from build123d import *

# Parameters (mm, degrees)
EXTRUDE_1_DEPTH     = 5
SKETCH_2_R          = 1.25
CUT_EXTRUDE_1_DEPTH = 7.5
SKETCH_3_R          = 1.25
CUT_EXTRUDE_2_DEPTH = 7.5
SKETCH_4_R          = 1.25
CUT_EXTRUDE_3_DEPTH = 76.013332148
SKETCH_5_R          = 0.75
CUT_EXTRUDE_4_DEPTH = 76.013332148
SKETCH_7_R          = 1.5
CUT_EXTRUDE_6_DEPTH = 76.013332148


with BuildPart() as part:
    # ｽｹｯﾁ1 → ﾎﾞｽ - 押し出し1 (new body)
    with BuildSketch(Plane.XY):
        Polygon((-29, 51), (-29, 0), (-23, 0), (-23, -3), (23, -3), (23, 0), (29, 0), (29, 51), (23, 51), (23, 59), (17, 59), (17, 69), (-17, 69), (-17, 59), (-23, 59), (-23, 51), align=None)
    extrude(amount=EXTRUDE_1_DEPTH)

    # ｽｹｯﾁ2 → ｶｯﾄ - 押し出し1 (cut)
    with BuildSketch(Plane(origin=(0, 59, 0), x_dir=(1, 0, 0), z_dir=(0, 1, 0))):
        with Locations(Location((-20, -2.5, 0), (0, 0, 270))):
            Circle(SKETCH_2_R)
        with Locations(Location((20, -2.5, 0), (0, 0, 270))):
            Circle(SKETCH_2_R)
    extrude(amount=-CUT_EXTRUDE_1_DEPTH, mode=Mode.SUBTRACT)

    # ｽｹｯﾁ3 → ｶｯﾄ - 押し出し2 (cut)
    with BuildSketch(Plane(origin=(0, 51, 0), x_dir=(1, 0, 0), z_dir=(0, 1, 0))):
        with Locations(Location((-26, -2.5, 0), (0, 0, 270))):
            Circle(SKETCH_3_R)
        with Locations(Location((26, -2.5, 0), (0, 0, 270))):
            Circle(SKETCH_3_R)
    cut_extrude_2 = extrude(amount=-CUT_EXTRUDE_2_DEPTH, mode=Mode.SUBTRACT)

    # ﾐﾗｰ1: ｶｯﾄ - 押し出し2 across plane
    add(cut_extrude_2.mirror(Plane.ZX.offset(25.5)), mode=Mode.SUBTRACT)

    # ｽｹｯﾁ4 → ｶｯﾄ - 押し出し3 (cut, through all)
    with BuildSketch(Plane(origin=(0, 0, 0), x_dir=(-1, 0, 0), z_dir=(0, 0, -1))):
        with Locations((-14.5, 66.5)):
            Circle(SKETCH_4_R)
        with Locations((14.5, 66.5)):
            Circle(SKETCH_4_R)
    extrude(amount=-CUT_EXTRUDE_3_DEPTH, mode=Mode.SUBTRACT)

    # ｽｹｯﾁ5 → ｶｯﾄ - 押し出し4 (cut, through all)
    with BuildSketch(Plane(origin=(0, 0, 0), x_dir=(-1, 0, 0), z_dir=(0, 0, -1))):
        with Locations((-17, 59)):
            Circle(SKETCH_5_R)
        with Locations((-23, 51)):
            Circle(SKETCH_5_R)
        with Locations((-23, 0)):
            Circle(SKETCH_5_R)
        with Locations((17, 59)):
            Circle(SKETCH_5_R)
        with Locations((23, 51)):
            Circle(SKETCH_5_R)
        with Locations((23, 0)):
            Circle(SKETCH_5_R)
    extrude(amount=-CUT_EXTRUDE_4_DEPTH, mode=Mode.SUBTRACT)

    # ｽｹｯﾁ7 → ｶｯﾄ - 押し出し6 (cut, through all)
    with BuildSketch(Plane.XY.offset(5)):
        with Locations((-26, 44)):
            Circle(SKETCH_7_R)
        with Locations(Location((-26, 7, 0), (0, 0, 180))):
            Circle(SKETCH_7_R)
        with Locations((-20, 52)):
            Circle(SKETCH_7_R)
        with Locations(Location((20, 52, 0), (0, 0, 180))):
            Circle(SKETCH_7_R)
        with Locations((26, 7)):
            Circle(SKETCH_7_R)
        with Locations(Location((26, 44, 0), (0, 0, 180))):
            Circle(SKETCH_7_R)
    extrude(amount=-CUT_EXTRUDE_6_DEPTH, mode=Mode.SUBTRACT)


solid = part.part
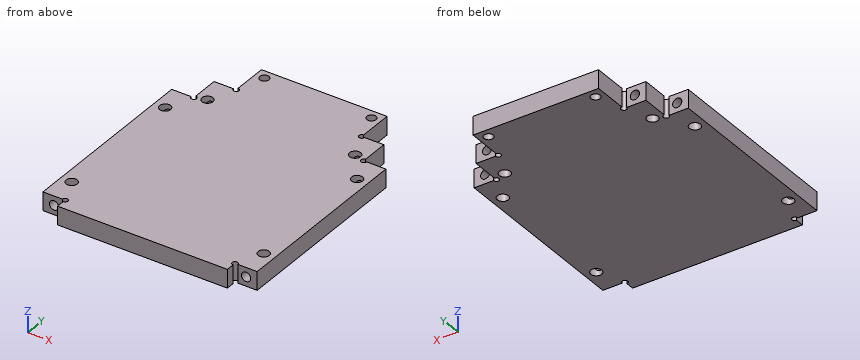
The listing builds one solid part. Answer for the finished solid, in the listing's coordinates (mm). Coordinates: 2 decimals unless noted, no trailing zeros. Order: outer loops, then holes, each group sorted by start corner. A loop starts at its lowest first (then second) coordinate and runs counter-clockwise, first axis right, second up. Notation, with made-up numbers: M -27,5.25 L 3,5.25 A31 cw 3,33.25 Z; hole C 48,-27.5 d2. An arc over 180 degrees is marked long. Use CSV: the item, a comma, the result in double quotes.
Q1. Given pin 1 Ø2.5 at (x, z) = (-21, 2.5) entering from +Y; pin 2 Ø2.5 at (x, y) = (-20, 52) entering from +Z (1 decimal); pin 3 Ø1.5 at (x, y) = (21, 7) entering from -Z; pin 4 Ø1.5 at (y, z) = (63.5, 1.5) entering from +X, each flat-ended and moving along its own axis, determine where each tip first touches the part or whether it passes through.
Here are the results:
pin 1,"y = 59"
pin 2,"through"
pin 3,"z = 0"
pin 4,"x = 17"
Q2. Section D-D (y = 63.5) is taken. Determine the outline of the cut face in (x, z).
Here are the results:
outline,"M -17,0 L 17,0 L 17,5 L -17,5 Z"
Q3. Section C-C (x = -20) is taken. Determine the outline of the cut face in (y, z).
Here are the results:
outline,"M -3,0 L 50.5,0 L 50.5,5 L -3,5 Z; M 53.5,0 L 59,0 L 59,1.25 L 53.5,1.25 Z; M 53.5,3.75 L 59,3.75 L 59,5 L 53.5,5 Z"
Q4. Section A-A (x = 26) is taken. Determine the outline of the cut face in (y, z).
Here are the results:
outline,"M 0,0 L 5.5,0 L 5.5,1.25 L 0,1.25 Z; M 0,3.75 L 5.5,3.75 L 5.5,5 L 0,5 Z; M 8.5,0 L 42.5,0 L 42.5,5 L 8.5,5 Z; M 45.5,0 L 51,0 L 51,1.25 L 45.5,1.25 Z; M 45.5,3.75 L 51,3.75 L 51,5 L 45.5,5 Z"
Q5. Section B-B (y = 44) is taken. Determine the outline of the cut face in (x, z).
Here are the results:
outline,"M -29,0 L -27.5,0 L -27.5,5 L -29,5 Z; M -24.5,0 L 24.5,0 L 24.5,5 L -24.5,5 Z; M 27.5,0 L 29,0 L 29,5 L 27.5,5 Z"
Q6. Straight lines are drawn through the part: L1, parallel to X at y = 66.5, z = 2.15; L2, parallel to Z at x = 26, y = 48.5; L3, parallel to X at y = 49.5, z = 2.5. For each, find the intervals that lie inside material, in ascending order.
Here are the results:
L1,"-17 to -15.75, -13.25 to 13.25, 15.75 to 17"
L2,"0 to 1.25, 3.75 to 5"
L3,"-29 to -27.25, -24.75 to 24.75, 27.25 to 29"
